Geometry check sheet. Reference: the model listing, model coordinates, mm. Face numbers are marked on the shaded views. A direction names the side the tool comes from. Give positions to 0.01 mm unless a question says otherwise; leave off trailing zeros. Write each loop counter-clockwise with the first axis right and the second up, starting at its lowest first coordinate (ties: lowest second). Pieces come first, ordered by that corner, then holes. Notation, with made-up numbers: (30, 21.5) -> (75, 21.5) arc R25 ccw to (75, 55.5) -> close; hole circle Ø1 at (44.5, -0.75). An arc over 180 degrees is marked (long way). One line per item, written item: value.
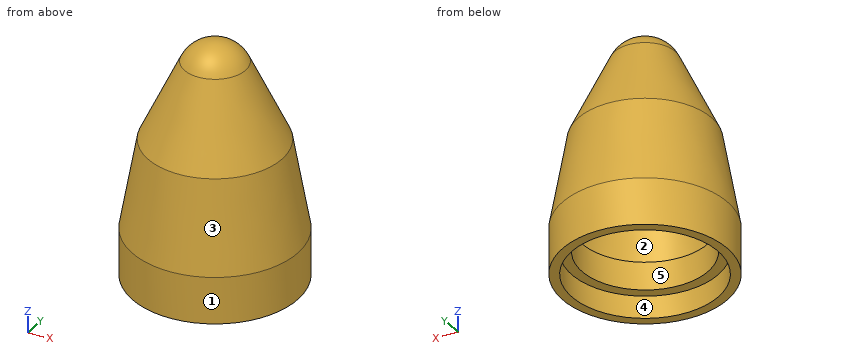
from build123d import *

# Parameters (mm, degrees)
F3_ANGLE = 90


with BuildPart() as f1:
    # F0 (on Top) → F1 (revolve)
    with BuildSketch(Plane.XY):
        with BuildLine():
            Line((0, 8.9), (0, 7.9))
            Line((0, 7.9), (2.4, 7.9))
            Line((2.4, 7.9), (2.4, 6.8))
            Line((2.4, 6.8), (5.4, 6.8))
            Line((5.4, 6.8), (5.4, 7.7508590184))
            Line((5.4, 7.7508590184), (14.092461206, 6.2356893905))
            Line((14.092461206, 6.2356893905), (21.86847149, 2.6096762451))
            Line((21.86847149, 2.6096762451), (24.1485125287, 0))
            Line((24.1485125287, 0), (25.1485125287, 0))
            ThreePointArc((25.1485125287, 0), (24.5807771156, 1.9478119615), (23.0553953206, 3.2855358927))
            Line((23.0553953206, 3.2855358927), (14.6574713698, 7.2015521436))
            Line((14.6574713698, 7.2015521436), (5.0250949202, 8.9))
            Line((5.0250949202, 8.9), (0, 8.9))
        make_face()
    revolve(axis=Axis((12.5827532146, 0, 0), (1, 0, 0)))


with BuildPart() as f1_1:
    # F3: moved
    add(f1.part.rotate(Axis((0, 0, 0), (0, -1, 0)), F3_ANGLE))


solid = f1_1.part
1) Tool access check on the marked faces 1 and 2. Record the directions out of +Z, -Z, +X, -X, +Y, -Y that give a thin tool (end or side, any length) a straight path to the whole face; none if there is none.
Verdict:
face 1: +Z, -Z
face 2: none
2) Scan lines: probe 1 along X at (y, z) = (0, 4.7); probe 2 along X at (y, z) = (0, 1.55). Record each from-to range of solid material in increasing order.
Verdict:
probe 1: -8.9 to -6.8, 6.8 to 8.9
probe 2: -8.9 to -7.9, 7.9 to 8.9
3) Mould release check, pull along X, two halves, no side actions. Record for the marked faces 3, 4 and 5: released by +X, released by -X, zero draft, split by the parting line, or undercut.
Verdict:
face 3: split by the parting line
face 4: undercut
face 5: undercut
4) Sectioned sample at A-A on z = 21.25. Record the cut outline in (x, y).
Verdict:
outline: circle Ø8.25 at (0, 0); hole circle Ø5.8 at (0, 0)
5) Depth check by flat-ended pin: pin 1 Ø1 at (y, z) = (-4, 10.5) entering from +X; pin 2 Ø10 at (y, z) = (-6, 11.5) entering from -X; pin 3 Ø3 at (x, z) = (-1, 17.5) entering from -Y. Enter the tip coordinate at first touch or a pass-through.
Verdict:
pin 1: x = 7.14
pin 2: x = -8.04
pin 3: y = -6.52
